from build123d import *

# Parameters (mm, degrees)
ESQUISSE1_W        = 45
ESQUISSE1_H        = 13
ESQUISSE1_R        = 2.13
ESQUISSE1_W_2      = 4
ESQUISSE1_H_2      = 7
BOSS_EXTRU_1_DEPTH = 4
CONG_1_R           = 2


with BuildPart() as part:
    # Esquisse1 → Boss.-Extru.1 (new body)
    with BuildSketch(Plane.XY):
        Rectangle(ESQUISSE1_W, ESQUISSE1_H)
        with Locations((-4.875, 2.32)):
            Circle(ESQUISSE1_R, mode=Mode.SUBTRACT)
        with Locations((4.875, 2.32)):
            Circle(ESQUISSE1_R, mode=Mode.SUBTRACT)
        with Locations((-17.5, 0)):
            Rectangle(ESQUISSE1_W_2, ESQUISSE1_H_2, mode=Mode.SUBTRACT)
        with Locations((17.5, 0)):
            Rectangle(ESQUISSE1_W_2, ESQUISSE1_H_2, mode=Mode.SUBTRACT)
    extrude(amount=BOSS_EXTRU_1_DEPTH)

    # Congé1
    cong_1_edges = [part.edges().sort_by_distance(p)[0] for p in [
        (-22.5, 6.5, 2),
        (22.5, 6.5, 2),
        (22.5, -6.5, 2),
        (-22.5, -6.5, 2),
    ]]
    fillet(cong_1_edges, radius=CONG_1_R)


solid = part.part
Build history of the part. All positions in model axes, mm. A direction names the side the tool comes from. Coordinates: 2 decimals unless noted, no trailing zeros. Order: outer loops, then holes, each group sorted by start corner. A loop starts at its lowest first (then second) coordinate and runs counter-clockwise, first axis right, second up. Notation, with made-up numbers: (-32.75, 68) - (-11.75, 68) arc R21 cw to (-11.75, 105) - close; hole circle Ø8 at (65, -26.75). An arc over 180 degrees is marked (long way). Write item = value, one per line. Start each with the question number.
1) Saw through at C-C on x = -17.5. Write the cut outline in (y, z), then the cut area to 3 significant figures.
2) Flat gauge pin, fed straight in: pin 1 Ø3.5 at (x, y) = (4.875, 2.32) entering from +Z. Where does the tip first touch, or does it go through?
3) 3-axis set-ups, long thin cutter, end or side, ignore diameter. For faces 5 (the face through (15.5, 0, 2)), 6 (the face through (-22.5, 0, 2)): which of +Z, -Z, +X, -X, +Y, -Y reach the whole face in a straight line?
4) Wall check: line 1 along X through (y, z) = (-3, 0.45); line 2 along Y through (x, z) = (-16, 1.6); line 3 along X through (y, z) = (2.75, 3.6). Give the ranges that are in metal, low to high. Write a range as from..to.
5) Saw through at B-B on z = 0.95. Write the cut outline in (x, y) (3 decimals).
6) Two-plate mould, pull along X, no slides. Class faces 1 (the face through (-18, 3.5, 2)), 2 (the face through (0, 0, 0)), 3 (the face through (21.9, -5.93, 2.03)), 4 (the face through (-21.93, 5.9, 2.03)): pulls with the +X half, pulls with the -X half, needs draft (parallel to the pull), parting line crosses it, or undercut.
7) Saw through at D-D on y = -3. Write the cut outline in (x, z), then the cut area to 3 significant figures.
8) Saw through at A-A on y = 2.32. Write the cut outline in (x, z) (3 decimals), then the cut area to 3 significant figures.
From the geometry:
q1.outline = (-6.5, 0) - (-3.5, 0) - (-3.5, 4) - (-6.5, 4) - close; (3.5, 0) - (6.5, 0) - (6.5, 4) - (3.5, 4) - close
q1.area = 24.0 mm^2
q2.pin_1 = through
q3.face_5 = +Z, -Z
q3.face_6 = +Z, -Z, -X, +Y, -Y
q4.line_1 = -22.5..-19.5, -15.5..15.5, 19.5..22.5
q4.line_2 = -6.5..-3.5, 3.5..6.5
q4.line_3 = -22.5..-19.5, -15.5..-6.96, -2.79..2.79, 6.96..15.5, 19.5..22.5
q5.outline = (-22.5, -4.5) arc R2 ccw to (-20.5, -6.5) - (20.5, -6.5) arc R2 ccw to (22.5, -4.5) - (22.5, 4.5) arc R2 ccw to (20.5, 6.5) - (-20.5, 6.5) arc R2 ccw to (-22.5, 4.5) - close; hole (-19.5, -3.5) - (-15.5, -3.5) - (-15.5, 3.5) - (-19.5, 3.5) - close; hole circle Ø4.26 at (-4.875, 2.32); hole circle Ø4.26 at (4.875, 2.32); hole (15.5, -3.5) - (19.5, -3.5) - (19.5, 3.5) - (15.5, 3.5) - close
q6.face_1 = undercut
q6.face_2 = needs draft
q6.face_3 = pulls with the +X half
q6.face_4 = pulls with the -X half
q7.outline = (-22.5, 0) - (-19.5, 0) - (-19.5, 4) - (-22.5, 4) - close; (-15.5, 0) - (15.5, 0) - (15.5, 4) - (-15.5, 4) - close; (19.5, 0) - (22.5, 0) - (22.5, 4) - (19.5, 4) - close
q7.area = 148 mm^2
q8.outline = (-22.5, 0) - (-19.5, 0) - (-19.5, 4) - (-22.5, 4) - close; (-15.5, 0) - (-7.005, 0) - (-7.005, 4) - (-15.5, 4) - close; (-2.745, 0) - (2.745, 0) - (2.745, 4) - (-2.745, 4) - close; (7.005, 0) - (15.5, 0) - (15.5, 4) - (7.005, 4) - close; (19.5, 0) - (22.5, 0) - (22.5, 4) - (19.5, 4) - close
q8.area = 114 mm^2
